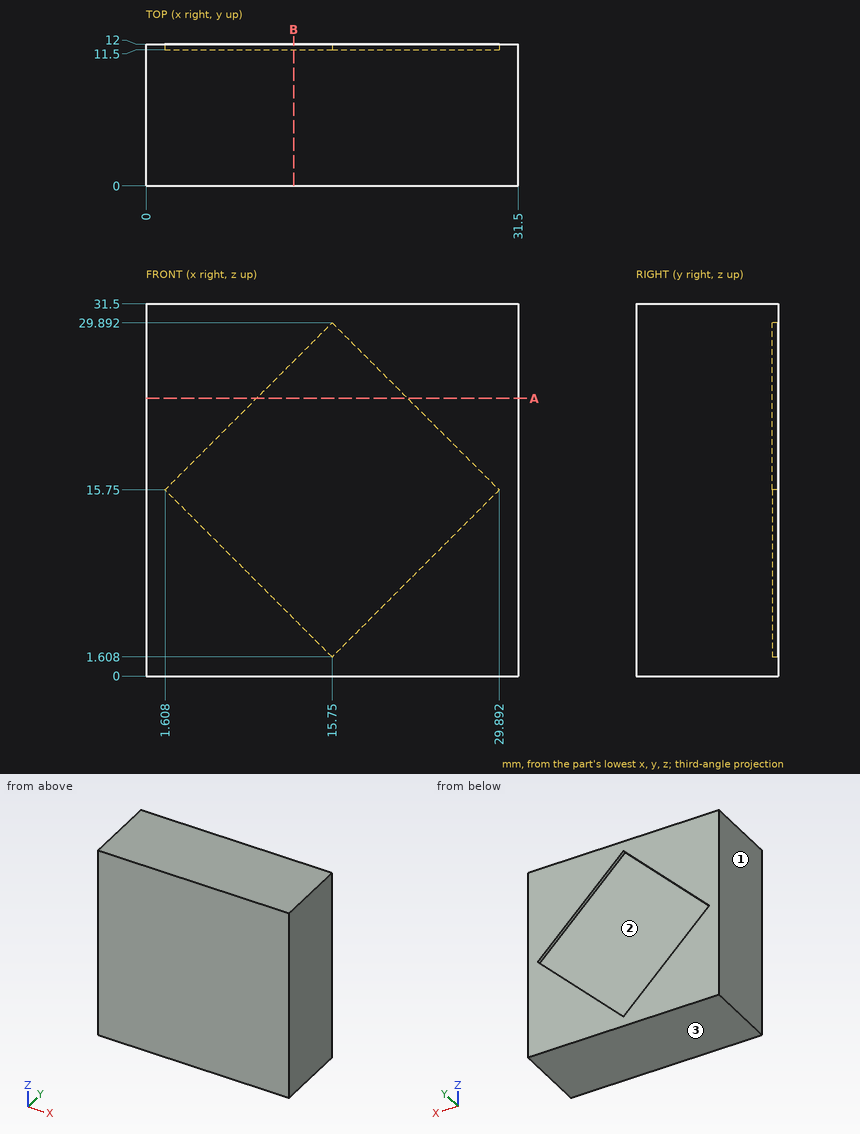
Can you work these out from the drawing? Everything is in mm from the part's minimum corner. Give positions to 0.01 mm unless a question says otherwise; leave off trailing zeros. Order: outer loops, then holes, each group sorted by start corner. A loop starts at its lowest first (then second) coordinate and runs counter-clockwise, first axis right, second up. Notation, with made-up numbers: M -20.75,87.5 L 36.25,87.5 A29 ccw 36.25,113.5 Z; hole C 77,4.5 d1. An arc over 180 degrees is marked long. Write item = value, one per line. Start each with the question number.
Q1. Will this pin go through, and if not, where does the flat tip stop? pin 1 Ø1.5 at (x, z) = (21.5, 17.5) entering from +Y.
Q2. Suppose I cut it at B-B (x = 12.5). Write out the boundary of the cut face in (y, z), plus the area to 3 significant figures.
Q3. I need wall thicknesses on probe 1 along Y at (x, z) = (15, 8). Which ranges of the line are inside material? Lowest first, please. Write a range as [from, to].
Q4. We'd pull the mould along X, two halves only. Please class the marked faces 1, 2 and 3: pulls with the +X half, pulls with the -X half, needs draft (parallel to the pull), parting line crosses it, or undercut.
Q5. Suppose I cut it at A-A (z = 23.5). Write out the boundary of the cut face in (x, y).
Check result:
q1.pin_1 = 11.5
q2.outline = M 0,0 L 12,0 L 12,4.86 L 11.5,4.86 L 11.5,26.64 L 12,26.64 L 12,31.5 L 0,31.5 Z
q2.area = 367 mm2
q3.probe_1 = [0, 11.5]
q4.face_1 = pulls with the -X half
q4.face_2 = undercut
q4.face_3 = needs draft
q5.outline = M 0,0 L 31.5,0 L 31.5,12 L 22.14,12 L 22.14,11.5 L 9.36,11.5 L 9.36,12 L 0,12 Z
